Check sheet for the drawn part. Datum: minimum x, y, z corner. Units: mm. A direction names the side the tool comes from. Coordinates: 2 decimals unless noted, no trailing zeros. Loops run counter-clockwise (first coordinate to the right, second up) from the corner with the lowest first, then second, coordinate; pieces in that order, holes last. Notation, with made-up numbers: (-9.5, 14.25) - (32.5, 14.25) arc R24 ccw to (32.5, 53.25) - close; hole circle Ø11 at (4.25, 62.5). An arc over 180 degrees is marked (long way). Answer as CSV lines item,"result". Start each with the question number.
1. Cross-section at B-B (z = 5.15). Enter the section's corners in (x, y), plus the area to 3 significant figures.
2. Cross-section at C-C (x = 7.5). Enter the section's corners in (y, z), plus the area to 3 significant figures.
3. Cross-section at A-A (x = 5.15). Enter the section's corners in (y, z), plus the area to 3 significant figures.
4. Gauge pin test, flat ends, axial feed: P1, Ø1, axis at x = 2, y = 1, coming from the -Z side; P2, Ø2, axis at x = 4.5, z = 4.5, coming from the -Y side. Record the tip position at first contact, or that the pin passes through.
5. Release check for a two-part mould opening along Z. For the marked faces 3, 4, 5 and 6 record: pulls with the +Z half, pulls with the -Z half, needs draft (parallel to the pull), parting line crosses it, or undercut.
6. Material ranges on line 1 (X direction, y = 2.4, z = 5.15); line 2 (X direction, y = 1.2, z = 5.15); line 3 (X direction, y = 0.1, z = 5.5), recorded low to high. Write a range as [from, to].
7. Cross-section at D-D (y = 1.55). Enter the section's corners in (x, z).
8. Set-up check for the marked faces 1 and 2: record each of +Z, -Z, +X, -X, +Y, -Y from which the full face is reachable in a straight line by a thin tool's end or side.
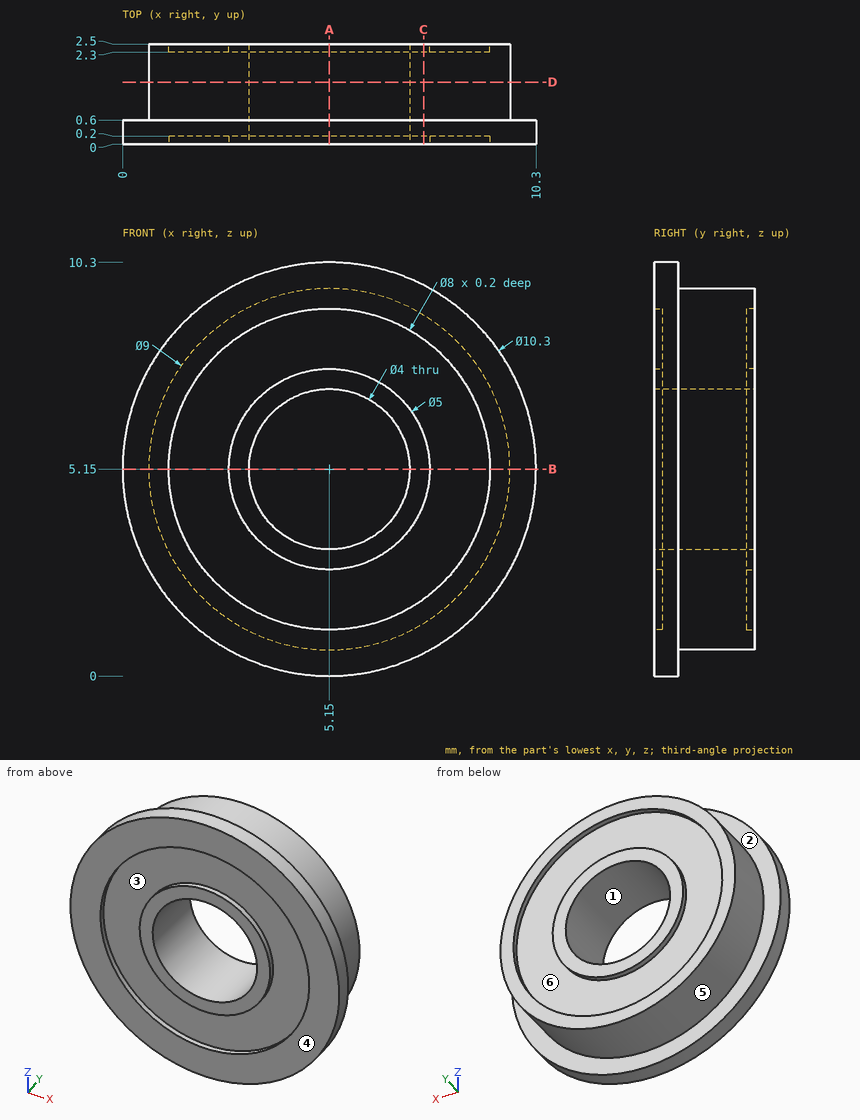
Values follow:
1,outline,"(0, 0) - (1.15, 0) - (1.15, 0.2) - (2.65, 0.2) - (2.65, 0) - (3.15, 0) - (3.15, 2.5) - (2.65, 2.5) - (2.65, 2.3) - (1.15, 2.3) - (1.15, 2.5) - (0.65, 2.5) - (0.65, 0.6) - (0, 0.6) - close; (7.15, 0) - (7.65, 0) - (7.65, 0.2) - (9.15, 0.2) - (9.15, 0) - (10.3, 0) - (10.3, 0.6) - (9.65, 0.6) - (9.65, 2.5) - (9.15, 2.5) - (9.15, 2.3) - (7.65, 2.3) - (7.65, 2.5) - (7.15, 2.5) - close"
1,area,"12.1 mm²"
2,outline,"(0, 0.57) - (0.6, 0.57) - (0.6, 1.31) - (2.5, 1.31) - (2.5, 1.91) - (2.3, 1.91) - (2.3, 4.3) - (2.5, 4.3) - (2.5, 6) - (2.3, 6) - (2.3, 8.39) - (2.5, 8.39) - (2.5, 8.99) - (0.6, 8.99) - (0.6, 9.73) - (0, 9.73) - (0, 8.39) - (0.2, 8.39) - (0.2, 6) - (0, 6) - (0, 4.3) - (0.2, 4.3) - (0.2, 1.91) - (0, 1.91) - close"
2,area,"18.2 mm²"
3,outline,"(0, 0) - (0.6, 0) - (0.6, 0.65) - (2.5, 0.65) - (2.5, 1.15) - (2.3, 1.15) - (2.3, 2.65) - (2.5, 2.65) - (2.5, 3.15) - (0, 3.15) - (0, 2.65) - (0.2, 2.65) - (0.2, 1.15) - (0, 1.15) - close; (0, 7.15) - (2.5, 7.15) - (2.5, 7.65) - (2.3, 7.65) - (2.3, 9.15) - (2.5, 9.15) - (2.5, 9.65) - (0.6, 9.65) - (0.6, 10.3) - (0, 10.3) - (0, 9.15) - (0.2, 9.15) - (0.2, 7.65) - (0, 7.65) - close"
3,area,"12.1 mm²"
4,P1,"stops at z = 0.86"
4,P2,"passes through"
5,face 3,"undercut"
5,face 4,"needs draft"
5,face 5,"parting line crosses it"
5,face 6,"undercut"
6,line 1,"x = [0.65, 1.15], [2.65, 3.15], [7.15, 7.65], [9.15, 9.65]"
6,line 2,"x = [0.65, 3.15], [7.15, 9.65]"
6,line 3,"x = [0.01, 1.17], [2.67, 3.18], [7.12, 7.63], [9.13, 10.29]"
7,outline,"circle Ø9 at (5.15, 5.15); hole circle Ø4 at (5.15, 5.15)"
8,face 1,"+Y, -Y"
8,face 2,"+Y"
